from build123d import *

# Parameters (mm, degrees)
F0_W     = 17.6831819117
F0_H     = 10.16
F2_R     = 12.7
F3_DEPTH = 6.35
F4_W     = 9.8243676867
F4_H     = 5.08
F5_DEPTH = 6.35
F7_R     = 0.9355774764


# Not quite as in the source:
# - a fillet or chamfer that OpenCascade refuses, or shapes differently, is made with other operations: its cross-section is extruded or revolved along the edge and cut away or added


with BuildPart() as f1:
    # F0 (on Front) → F1 (revolve)
    with BuildSketch(Plane.XZ):
        with Locations((8.8415909559, 52.07)):
            Rectangle(F0_W, F0_H)
        with BuildLine():
            Line((0, 46.99), (0, 0))
            Line((0, 0), (19.05, 0))
            Line((19.05, 0), (19.05, 9.525))
            add(Edge.make_bspline(
                [(19.05, 9.525), (17.1376126861, 14.5770803043), (12.2594277566, 14.0530870359), (15.8311377158, 27.1771005404), (4.8442118801, 31.8163009505), (10.984866263, 42.7056935759), (14.4496818428, 44.7679251006), (17.6831819117, 46.99)],
                knots=[0, 0, 0, 0, 0.192461159, 0.3996068615, 0.6001290124, 0.8022738887, 1, 1, 1, 1], degree=3))
            Line((17.6831819117, 46.99), (0, 46.99))
        make_face()
    revolve(axis=Axis((0, 0, 28.575), (0, 0, 1)))

    # F2 (on face) → F3 (cut)
    with BuildSketch(Plane.XY.offset(57.15)):
        Circle(F2_R)
    extrude(amount=-F3_DEPTH, mode=Mode.SUBTRACT)

    # F4 (on face) → F5 (cut)
    with BuildSketch(Plane.XY.offset(57.15)):
        with Locations((15.24, 0)):
            Rectangle(F4_W, F4_H)
        Polygon((6.8624042447, 8.125441191), (9.8483533263, 4.0156348596), (17.7964337439, 9.7902532989), (14.8104846622, 13.9000596303), align=None)
        Polygon((0.7757871558, 10.6072400206), (5.6071542586, 9.0374336892), (8.6430508328, 18.3809625961), (3.81168373, 19.9507689275), align=None)
        Polygon((-5.6071542586, 9.0374336892), (-0.7757871558, 10.6072400206), (-3.81168373, 19.9507689275), (-8.6430508328, 18.3809625961), align=None)
        Polygon((-9.8483533263, 4.0156348596), (-6.8624042447, 8.125441191), (-14.8104846622, 13.9000596303), (-17.7964337439, 9.7902532989), align=None)
        with Locations((-15.24, 0)):
            Rectangle(F4_W, F4_H)
        Polygon((-6.8624042447, -8.125441191), (-9.8483533263, -4.0156348596), (-17.7964337439, -9.7902532989), (-14.8104846622, -13.9000596303), align=None)
        Polygon((-0.7757871558, -10.6072400206), (-5.6071542586, -9.0374336892), (-8.6430508328, -18.3809625961), (-3.81168373, -19.9507689275), align=None)
        Polygon((5.6071542586, -9.0374336892), (0.7757871558, -10.6072400206), (3.81168373, -19.9507689275), (8.6430508328, -18.3809625961), align=None)
        Polygon((9.8483533263, -4.0156348596), (6.8624042447, -8.125441191), (14.8104846622, -13.9000596303), (17.7964337439, -9.7902532989), align=None)
    extrude(amount=-F5_DEPTH, mode=Mode.SUBTRACT)

    # F6: chamfer of 5.08 on 1 edges, made by hand

    # F6_s1 → F6_t2 (revolve, cut)
    with BuildSketch(Plane.XZ):
        with BuildLine():
            Line((13.7794309142, 44.1484930415), (17.7734832624, 52.1998472193))
            Line((17.7734832624, 52.1998472193), (17.8750832624, 52.1998472193))
            ThreePointArc((17.8750832624, 52.1998472193), (17.7847819117, 49.5949236096), (17.7847819117, 46.99))
            Line((17.7847819117, 46.99), (17.7407244212, 46.90626578))
            ThreePointArc((17.7407244212, 46.90626578), (15.7475972656, 45.5454980697), (13.8409013181, 44.0675983603))
            Line((13.8409013181, 44.0675983603), (13.7794309142, 44.1484930415))
        make_face()
    revolve(axis=Axis((0, 0, 46.99), (0, 0, 1)), mode=Mode.SUBTRACT)

    # F7 (on Front) → F8 (revolve, cut)
    with BuildSketch(Plane.XZ):
        with Locations((19.0286766738, 5.0287479535)):
            Circle(F7_R)
    revolve(axis=Axis((0, 0, 5.0287479535), (0, 0, 1)), mode=Mode.SUBTRACT)


solid = f1.part
Here's how the part is built. I have some questions about the finished solid (model axes, mm). A direction names the side the tool comes from. Round coordinates to 2 decimals unless told otherwise and drop trailing zeros. One line per question, with ' | ' between items. Start each with the question number.
Q1. Please list where these lines run through material, in increasing order: line 1 (Z direction, x = 11, y = 1.5); line 2 (Z direction, x = -14, y = -8); line 3 (X direction, y = -15, z = 55.5). Write a range as [from, to].
Q2. Will these pins go through, and if not, where does the flat tip stop? pin 1 (4 mm diameter, centred on x = -9, z = 14, fed in from -Y); pin 2 (1.5 mm diameter, centred on x = -14, z = 55, fed in from +Y); pin 3 (12 mm diameter, centred on y = -10.5, z = 13, fed in from -X).
Q3. For faces 1 (the flat face through (-13.577, -6.724, 54.019)), 2 (the flat face through (7.053, -13.488, 54.019)), 3 (the flat face through (-7.053, 13.488, 54.019)), 4 (the conical face through (13.457, 4.238, 44.811)), 5 (the flat face through (15, 2.54, 54)), which set-ups out of +Z, -Z, +X, -X, +Y, -Y let a thin tool reach every point of the face, with its end or its side?
Q4. We'd pull the mould along Y, two halves only. Please class faces 6 (the cylindrical face through (-15.12, -11.59, 7.77)), 7 (the cylindrical face through (12.072, -3.944, 54.019)), 8 (the flat face through (15, -5, 57.15)), 9 (the cylindrical face through (12.085, 3.905, 54.019)): +Y half, -Y half, draft (parallel to the pull), parting line (faces both ways), or undercut.
Response values:
1) line 1: z = [0, 28.77], [41.74, 50.8] | line 2: z = [0, 14.05], [48.88, 50.8] | line 3: x = [-9.36, -7.54], [-2.2, 2.2], [7.54, 9.36]
2) pin 1: stops at y = -15.77 | pin 2: stops at y = 7.58 | pin 3: stops at x = -18.21
3) face 1: +Z | face 2: +Z, -Y | face 3: +Z, +Y | face 4: none | face 5: +Z, +X, -X
4) face 6: parting line | face 7: undercut | face 8: draft | face 9: undercut
